Source: CAD feature listing. Evaluate the final solid. Frame: model axes, mm. A direction names the side the tool comes from. Give positions to 0.01 mm unless a question says otherwise; leave off trailing zeros. Order: outer loops, then holes, each group sorted by start corner. A loop starts at its lowest first (then second) coordinate and runs counter-clockwise, first axis right, second up. Notation, with made-up numbers: (4, -39) - (32, -39) arc R30 ccw to (32, -8) - close; hole circle Ø10 at (19, 42.5). An arc over 180 degrees is marked (long way). Use CSV: the item, a comma, the result in double quotes.
```python
from build123d import *

# Parameters (mm, degrees)
SKETCH_1_R          = 4
EXTRUDE_1_DEPTH     = 24
SKETCH_2_W          = 72
SKETCH_2_H          = 16
CUT_EXTRUDE_1_DEPTH = 107.451867057
SKETCH_3_R          = 8
CUT_EXTRUDE_2_DEPTH = 8
SKETCH_5_R          = 32
EXTRUDE_2_DEPTH     = 60
SKETCH_6_R          = 24
CUT_EXTRUDE_3_DEPTH = 35
CUT_EXTRUDE_4_DEPTH = 15
SKETCH_8_R          = 6.5
CUT_EXTRUDE_5_DEPTH = 86
SKETCH_9_R          = 11
CUT_EXTRUDE_6_DEPTH = 86
SKETCH_10_W         = 22
SKETCH_10_H         = 21.722562354
CUT_EXTRUDE_7_DEPTH = 38
RIB_8_REACH         = 116.07
SKETCH_12_WALL_W    = 293.316673134
SKETCH_12_WALL_H    = 12


with BuildPart() as part:
    # 草图1 → 凸台-拉伸1 (new body)
    with BuildSketch(Plane(origin=(0, 0, 0), x_dir=(1, 0, 0), z_dir=(0, 1, 0))):
        with BuildLine():
            Line((51, 40), (-51, 40))
            ThreePointArc((-51, 40), (-61.606601718, 35.606601718), (-66, 25))
            Line((-66, 25), (-66, -25))
            ThreePointArc((-66, -25), (-61.606601718, -35.606601718), (-51, -40))
            Line((-51, -40), (51, -40))
            ThreePointArc((51, -40), (61.606601718, -35.606601718), (66, -25))
            Line((66, -25), (66, 25))
            ThreePointArc((66, 25), (61.606601718, 35.606601718), (51, 40))
        make_face()
        with Locations(Location((-50, 24, 0), (0, 0, 270))):
            Circle(SKETCH_1_R, mode=Mode.SUBTRACT)
        with Locations(Location((50, 24, 0), (0, 0, 270))):
            Circle(SKETCH_1_R, mode=Mode.SUBTRACT)
        with Locations(Location((50, -24, 0), (0, 0, 270))):
            Circle(SKETCH_1_R, mode=Mode.SUBTRACT)
        with Locations(Location((-50, -24, 0), (0, 0, 270))):
            Circle(SKETCH_1_R, mode=Mode.SUBTRACT)
    extrude(amount=EXTRUDE_1_DEPTH)

    # 草图2 → 切除-拉伸1 (cut, through all)
    with BuildSketch(Plane.XY.offset(40)):
        Rectangle(SKETCH_2_W, SKETCH_2_H)
    extrude(amount=-CUT_EXTRUDE_1_DEPTH, mode=Mode.SUBTRACT)

    # 草图3 → 切除-拉伸2 (cut)
    with BuildSketch(Plane(origin=(0, 24, 0), x_dir=(1, 0, 0), z_dir=(0, 1, 0))):
        with Locations(Location((-50, 24, 0), (0, 0, 270))):
            Circle(SKETCH_3_R)
        with Locations(Location((50, 24, 0), (0, 0, 270))):
            Circle(SKETCH_3_R)
        with Locations(Location((50, -24, 0), (0, 0, 270))):
            Circle(SKETCH_3_R)
        with Locations(Location((-50, -24, 0), (0, 0, 270))):
            Circle(SKETCH_3_R)
    extrude(amount=-CUT_EXTRUDE_2_DEPTH, mode=Mode.SUBTRACT)

    # 草图5 → 凸台-拉伸2 (add)
    with BuildSketch(Plane(origin=(0, 24, 0), x_dir=(1, 0, 0), z_dir=(0, 1, 0))):
        with Locations(Location((0, 0, 0), (0, 0, 90))):
            Circle(SKETCH_5_R)
    extrude(amount=EXTRUDE_2_DEPTH)

    # 草图6 → 切除-拉伸3 (cut)
    with BuildSketch(Plane(origin=(0, 84, 0), x_dir=(1, 0, 0), z_dir=(0, 1, 0))):
        with Locations(Location((0, 0, 0), (0, 0, 270))):
            Circle(SKETCH_6_R)
    extrude(amount=-CUT_EXTRUDE_3_DEPTH, mode=Mode.SUBTRACT)

    # 草图7 → 切除-拉伸4 (cut)
    with BuildSketch(Plane(origin=(0, 49, 0), x_dir=(1, 0, 0), z_dir=(0, 1, 0))):
        Polygon((6.5, -12), (-6.5, -12), (-6.5, 0), (-13, 0), (-13, 10), (13, 10), (13, 0), (6.5, 0), align=None)
    extrude(amount=-CUT_EXTRUDE_4_DEPTH, mode=Mode.SUBTRACT)

    # 草图8 → 切除-拉伸5 (cut)
    with BuildSketch(Plane(origin=(0, 49, 0), x_dir=(1, 0, 0), z_dir=(0, 1, 0))):
        with Locations(Location((0, -12, 0), (0, 0, 180))):
            Circle(SKETCH_8_R)
    extrude(amount=-CUT_EXTRUDE_5_DEPTH, mode=Mode.SUBTRACT)

    # 草图9 → 切除-拉伸6 (cut)
    with BuildSketch(Plane.XY.offset(40)):
        with Locations((0, 66)):
            Circle(SKETCH_9_R)
    extrude(amount=-CUT_EXTRUDE_6_DEPTH, mode=Mode.SUBTRACT)

    # 草图10 → 切除-拉伸7 (cut)
    with BuildSketch(Plane.XY.offset(40)):
        with Locations((0, 76.861281177)):
            Rectangle(SKETCH_10_W, SKETCH_10_H)
    extrude(amount=-CUT_EXTRUDE_7_DEPTH, mode=Mode.SUBTRACT)

    # 草图12 wall → 筋8 (add, up to next)
    with BuildSketch(Plane(origin=(-48.467514941, 50.275944325, 0), x_dir=(0.555033040636, 0.831828301876, 0), z_dir=(-0.831828301876, 0.555033040636, 0)), mode=Mode.PRIVATE) as rib_8_sk1:
        Rectangle(SKETCH_12_WALL_W, SKETCH_12_WALL_H)
    rib_8_tool1 = extrude(rib_8_sk1.sketch, amount=-RIB_8_REACH, mode=Mode.PRIVATE) - part.part
    rib_8 = rib_8_tool1.solids().sort_by_distance((-48.467514941, 50.275944325, 0))[0]
    add(rib_8)

    # 镜向2: 筋8 across plane
    add(rib_8.mirror(Plane(origin=(0, 0, 0), x_dir=(0, 0, 1), z_dir=(1, 0, 0))))


solid = part.part
```
Item 1: Section C-C on z = -34. Return the cut outline in (x, y).
Filled in:
outline,"(-63, 0) - (-36, 0) - (-36, 8) - (36, 8) - (36, 0) - (63, 0) - (63, 24) - (-63, 24) - close"
Item 2: Set-up query: faces 1 (the flat face through (48, 16, -28)), 2 (the cylindrical face through (47.6, 7.9, -27.2)). Return all of +Z, -Z, +X, -X, +Y, -Y with unobstructed straight access to the full face (end or side cutting, diameter ignored); none if empty.
Filled in:
face 1,"+Y"
face 2,"+Y, -Y"
Item 3: Section D-D on y = 36. Return the cut outline in (x, z).
Filled in:
outline,"(-57.99, -6) - (-31.43, -6) arc R32 ccw to (31.43, -6) - (57.99, -6) - (57.99, 6) - (31.43, 6) arc R32 ccw to (-31.43, 6) - (-57.99, 6) - close; hole (-13, -10) - (13, -10) - (13, 0) - (6.5, 0) - (6.5, 12) arc R6.5 ccw to (-6.5, 12) - (-6.5, 0) - (-13, 0) - close"
Item 4: Section A-A on y = 18.5. Return the cut outline in (x, z), then the cut area to 3 significant figures.
Filled in:
outline,"(-66, -25) arc R15 ccw to (-51, -40) - (51, -40) arc R15 ccw to (66, -25) - (66, 25) arc R15 ccw to (51, 40) - (-51, 40) arc R15 ccw to (-66, 25) - close; hole circle Ø16 at (-50, -24); hole circle Ø16 at (-50, 24); hole circle Ø13 at (0, 12); hole circle Ø16 at (50, -24); hole circle Ø16 at (50, 24)"
area,"9,430 mm2"
Item 5: Section B-B on z = 26.5. Count the separate pieces of the cut face and the enclosed holes in it, then the cut area to 3 significant figures.
Filled in:
separate pieces,"3"
enclosed holes,"0"
area,"3,710 mm2"
Item 6: First-contact query: pin 1 (5 mm diameter, centred on x = -52, z = -22, fed in from +Y); pin 2 (12 mm diameter, centred on x = -52.5, y = 45.5, fed in from +Z); pin 3 (17.5 mm diameter, centred on x = -5.5, z = -2.5, fed in from +Y). Flat tips, straight axial feed; report the tip coordinate or a pass-through.
Filled in:
pin 1,"stops at y = 16"
pin 2,"stops at z = 6"
pin 3,"stops at y = 49"
Item 7: Mould query, pull axis Z, two halves, no side actions, for faces 3 (the flat face through (10, 42, 0)), 4 (the flat face through (40, 43, -6)), 5 (the flat face through (-51, 0, -1)). Classes: released by +Z, released by -Z, zero draft, split by the parting line, or undercut.
Filled in:
face 3,"undercut"
face 4,"released by -Z"
face 5,"zero draft"
Item 8: Material intervals for line 1 (Z direction, x = 50, y = 5.25); line 2 (X direction, y = 12, z = 24); line 3 (X direction, y = 15, z = 22), sorted ascending. Write a range as from..to.
Filled in:
line 1,"z = -40..-28, -20..20, 28..40"
line 2,"x = -66..-54, -46..46, 54..66"
line 3,"x = -66..-53.46, -46.54..46.54, 53.46..66"
